Here's how the part is built. I have some questions about the finished solid (model axes, mm). Face numbers are marked on the shaded views. A direction names the side the tool comes from. Give positions to 0.01 mm unless a question says otherwise; leave off trailing zeros. Loops run counter-clockwise (first coordinate to the right, second up) from the corner with the lowest first, then second, coordinate; pieces in that order, holes last. Notation, with made-up numbers: (38.25, 14.25) - (55.25, 14.25) arc R6 ccw to (55.25, 21.25) - close; hole circle Ø11 at (78.5, -37). An arc over 180 degrees is marked (long way). Use a Markdown table: item, result.
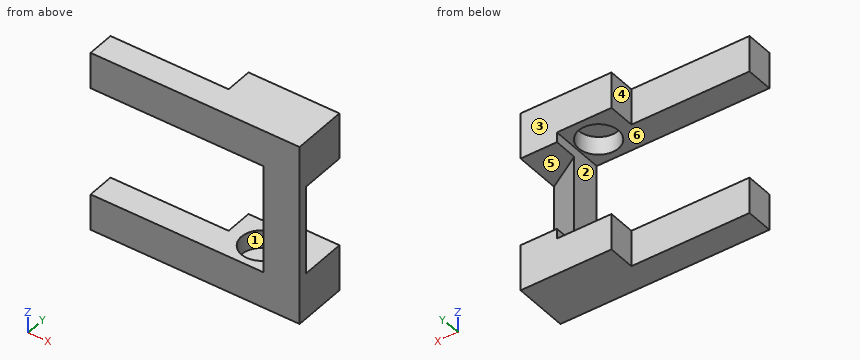
from build123d import *

# Parameters (mm, degrees)
IZIM1_W                          = 280
IZIM1_H                          = 100
IZIM1_W_2                        = 240
IZIM1_H_2                        = 60
Y_KSEKLIK_EKSTR_ZYON1_DEPTH      = 30
IZIM4_R                          = 11
KES_EKSTR_ZYON1_DEPTH            = 40
IZIM5_W                          = 65
IZIM5_H                          = 15
KES_EKSTR_ZYON2_DEPTH            = 119
KES_EKSTR_ZYON3_DEPTH            = 24.5
Y_KSEKLIK_EKSTR_ZYON4_DEPTH      = 8
Y_KSEKLIK_EKSTR_ZYON4_DEPTH_BACK = 1
IZIM13_R                         = 7.75
KES_EKSTR_ZYON4_DEPTH            = 18
IZIM14_W                         = 170.35585657
IZIM14_H                         = 104.641272027
KES_EKSTR_ZYON6_DEPTH            = 136


with BuildPart() as part:
    # Çizim1 → Yükseklik-Ekstrüzyon1 (new body)
    with BuildSketch(Plane(origin=(0, 0, 0), x_dir=(1, 0, 0), z_dir=(0, 1, 0))):
        with Locations((120, 30)):
            Rectangle(IZIM1_W, IZIM1_H)
        with Locations((120, 30)):
            Rectangle(IZIM1_W_2, IZIM1_H_2, mode=Mode.SUBTRACT)
    extrude(amount=Y_KSEKLIK_EKSTR_ZYON1_DEPTH)

    # Çizim4 → Kes-Ekstrüzyon1 (cut, symmetric)
    with BuildSketch(Plane.XY.offset(-30)):
        with Locations((228.036930768, 15)):
            Circle(IZIM4_R)
        with Locations((16.579541137, 15)):
            Circle(IZIM4_R)
        with Locations((95.469880506, 15)):
            Circle(IZIM4_R)
    extrude(amount=KES_EKSTR_ZYON1_DEPTH, both=True, mode=Mode.SUBTRACT)

    # Çizim5 → Kes-Ekstrüzyon2 (cut)
    with BuildSketch(Plane.XY.offset(20)):
        with Locations((177.478221097, 22.5)):
            Rectangle(IZIM5_W, IZIM5_H)
    extrude(amount=-KES_EKSTR_ZYON2_DEPTH, mode=Mode.SUBTRACT)

    # Çizim6 → Kes-Ekstrüzyon3 (cut, symmetric)
    with BuildSketch(Plane.XY.offset(-30)):
        Polygon((260, 31.552276972), (234.133246527, 31.552276972), (234.359911555, 20.467639669), (260, 4.801073138), align=None)
    extrude(amount=KES_EKSTR_ZYON3_DEPTH, both=True, mode=Mode.SUBTRACT)

    # Çizim10 → Yükseklik-Ekstrüzyon4 (add, two sides: drawn at the far end of the back side and taken through both)
    with BuildSketch(Plane(origin=(0, 22, 0), x_dir=(1, 0, 0), z_dir=(0, 1, 0)).offset(-Y_KSEKLIK_EKSTR_ZYON4_DEPTH_BACK)):
        Polygon((55.057032044, 60), (144.978221097, 21.175943648), (144.978221097, 60), align=None)
    extrude(amount=Y_KSEKLIK_EKSTR_ZYON4_DEPTH + Y_KSEKLIK_EKSTR_ZYON4_DEPTH_BACK)

    # Çizim13 → Kes-Ekstrüzyon4 (cut)
    with BuildSketch(Plane(origin=(0, 0, -80), x_dir=(-1, 0, 0), z_dir=(0, 0, -1))):
        with Locations((-16.579541137, 15)):
            Circle(IZIM13_R)
    extrude(amount=-KES_EKSTR_ZYON4_DEPTH, mode=Mode.SUBTRACT)

    # Çizim14 → Kes-Ekstrüzyon6 (cut)
    with BuildSketch(Plane(origin=(0, 30, 0), x_dir=(1, 0, 0), z_dir=(0, 1, 0))):
        with Locations((59.800292812, 32.320636013)):
            Rectangle(IZIM14_W, IZIM14_H)
    extrude(amount=-KES_EKSTR_ZYON6_DEPTH, mode=Mode.SUBTRACT)


solid = part.part
(1) We'd pull the mould along Y, two halves only. Please class the marked faces 1, 2 and 3: pulls with the +Y half, pulls with the -Y half, needs draft (parallel to the pull), parting line crosses it, or undercut.
A:
| item | result |
|---|---|
| face 1 | undercut |
| face 2 | needs draft |
| face 3 | pulls with the +Y half |
(2) Will these pins go through, and if not, where does the flat tip stop? pin 1 (16 mm diameter, centred on x = 180, z = -66.5, fed in from +Y); pin 2 (7.5 mm diameter, centred on y = 19, z = 6, fed in from -X); pin 3 (2 mm diameter, centred on y = 18.5, z = -33.5, fed in from +X); pin 4 (15 mm diameter, centred on y = 18.5, z = -37.5, fed in from -X).
A:
| item | result |
|---|---|
| pin 1 | y = 15 |
| pin 2 | x = 209.98 |
| pin 3 | through |
| pin 4 | x = 240 |
(3) On a 3-axis mill with a long thin cutter (end or side, diameter ignored), from which of +Z, -Z, +X, -X, +Y, -Y can I reach the whole of each face in a straight line? I mean the marked faces 4, 5 and 6. Say none if no direction works.
A:
| item | result |
|---|---|
| face 4 | +Z, -Z, -X, +Y |
| face 5 | +X, +Y |
| face 6 | -X, +Y, -Y |
(4) If I drill on line 1 (Z direction, x = 249.5, y = 15.25); line 2 (Z direction, x = 215.5, y = 9.5); line 3 (X direction, y = 22, z = -56.5), over which ranges is the centre line in solid material (lowest first)?
A:
| item | result |
|---|---|
| line 1 | -80 to -54.5, -5.5 to 20 |
| line 2 | -80 to -60, 0 to 20 |
| line 3 | 240 to 260 |
(5) Suppose I cut it at A-A on z = 4. Write out the boundary of the cut face in (x, y).
A:
| item | result |
|---|---|
| outline | (144.98, 0) - (260, 0) - (260, 30) - (209.98, 30) - (209.98, 15) - (144.98, 15) - close; hole circle Ø22 at (228.04, 15) |
(6) Suppose I cut it at D-D on z = -18. Write out the boundary of the cut face in (x, y), plus the area to 3 significant figures.
A:
| item | result |
|---|---|
| outline | (240, 0) - (260, 0) - (260, 4.8) - (240, 17.02) - close |
| area | 218 mm2 |
(7) Suppose I cut it at C-C on y = 9.25. Write out the boundary of the cut face in (x, z).
A:
| item | result |
|---|---|
| outline | (144.98, -80) - (260, -80) - (260, -54.5) - (252.72, -54.5) - (252.72, -5.5) - (260, -5.5) - (260, 20) - (144.98, 20) - (144.98, 0) - (218.66, 0) - (218.66, 10) - (237.41, 10) - (237.41, 0) - (240, 0) - (240, -60) - (237.41, -60) - (237.41, -70) - (218.66, -70) - (218.66, -60) - (144.98, -60) - close |
(8) Suppose I cut it at B-B on x = 187. Write out the boundary of the cut face in (y, z).
A:
| item | result |
|---|---|
| outline | (0, -80) - (15, -80) - (15, -60) - (0, -60) - close; (0, 0) - (15, 0) - (15, 20) - (0, 20) - close |
